Build history of the part. All positions in model axes, mm. Coordinates: 2 decimals unless noted, no trailing zeros. Loops run counter-clockwise (first coordinate to the right, second up) from the corner with the lowest first, then second, coordinate; pieces in that order, holes last.
Item 1: Drill centre lines: line 1 along X through (y, z) = (77, 1.65); line 2 along X through (y, z) = (-5.5, 1); line 3 along X through (y, z) = (26, 1.6). Where is each one in solid material? Low to high.
Item 2: Cut at A-A (z = 1.25). Count the separate pieces of the cut face and the enclosed holes in it, and give its area (3 significant figures).
Item 3: Cut at B-B (x = 2). List the corners of the cut face in (y, z).
Item 4: Flat gauge pins, fed straight in: pin 1 (1 mm diameter, centred on x = 28.5, z = 1.5, fed in from -Y); pin 2 (1 mm diameter, centred on x = -40, z = 0.5, fed in from -Y) (3 decimals); pin 3 (1 mm diameter, centred on x = 48.5, z = 1, fed in from -Y). Where does each tip first touch, or does it go through?
Item 5: Cut at C-C (y = 5). List the corners of the cut face in (x, z).
from build123d import *

# Parameters (mm, degrees)
F0_R     = 1.4
F1_DEPTH = 2
F3_DEPTH = 2.001
F4_R     = 3
F5_R     = 3
F7_DEPTH = 2.001


with BuildPart() as f1:
    # F0 (on Top) → F1 (new body)
    with BuildSketch(Plane.XY):
        Polygon((64.72135955, -47.0228201834), (0, 142.2155100196), (-64.72135955, -47.0228201834), (0, 0), align=None)
        with Locations((-34, 25)):
            Circle(F0_R, mode=Mode.SUBTRACT)
        with Locations((34, 25)):
            Circle(F0_R, mode=Mode.SUBTRACT)
        with Locations((-17, 53.2155100196)):
            Circle(F0_R, mode=Mode.SUBTRACT)
        with Locations((-17, 77.2155100196)):
            Circle(F0_R, mode=Mode.SUBTRACT)
        with Locations((17, 53.2155100196)):
            Circle(F0_R, mode=Mode.SUBTRACT)
        with Locations((17, 77.2155100196)):
            Circle(F0_R, mode=Mode.SUBTRACT)
    extrude(amount=F1_DEPTH)

    # F2 (on face) → F3 (cut, through all)
    with BuildSketch(Plane.XY.offset(2)):
        Polygon((-11.72135955, -5.0228201834), (-46.72135955, -5.0228201834), (-47.4053791086, -7.0228201834), (-14.4741233909, -7.0228201834), align=None)
        Polygon((-12.4188465721, -9.0228201834), (-24.4188465721, -9.0228201834), (-26.4198078873, -10.9094650687), (-15.0155904826, -10.9094650687), align=None)
        Polygon((-23.72135955, -13.0228201834), (-50.72135955, -13.0228201834), (-51.2508899541, -14.5711104259), (-25.8523982474, -14.5711104259), align=None)
        Polygon((-54.6096456252, -17.4572506108), (-55.1764262564, -19.1144565314), (-45.8653729736, -19.1144565314), (-44.7456995673, -17.4572506108), align=None)
        Polygon((-36.183078901, -21.7685099146), (-52.9450522033, -21.7685099146), (-53.5922657988, -23.6608932166), (-38.7877210645, -23.6608932166), align=None)
        Polygon((-57.329058215, -25.4085220489), (-57.8811639638, -27.0228201834), (-51.9252746689, -27.0915274002), (-50.8447687747, -25.4085220489), align=None)
        Polygon((-42.8185183528, -25.398144593), (-49.1967415728, -25.398144593), (-50.3631159663, -27.0228201834), (-44.4640927017, -27.0228201834), align=None)
        Polygon((-34.9575470313, -25.398144593), (-39.6975811287, -25.398144593), (-41.5776334703, -27.0228201834), (-37.1937211406, -27.0228201834), align=None)
        Polygon((-46.72135955, -29.0228201834), (-54.72135955, -29.0228201834), (-55.3310927131, -30.8056147116), (-49.1751657065, -30.8056147116), align=None)
        Polygon((-59.9332226396, -33.0228201834), (-60.6172421983, -35.0228201834), (-58.1569412289, -35.0228201834), (-57.0628715088, -33.0228201834), align=None)
        Polygon((-52.0519517882, -9.9788275021), (-52.6991653837, -11.8712108041), (-38.9741415612, -11.8712108041), (-37.5880427095, -9.9788275021), align=None)
        Polygon((-32.9459308027, -19.1144565314), (-26.3087923894, -19.1144565314), (-24.3671516029, -17.7037719259), (-31.0042900162, -17.7037719259), align=None)
        Polygon((-35.6436006209, -17.440581688), (-43.3317036365, -17.440581688), (-44.5420111982, -19.1144565314), (-37.288930104, -19.1144565314), align=None)
        Polygon((-51.8852360547, -33.0228201834), (-54.9353141808, -33.0228201834), (-56.3333206621, -35.0228201834), (-53.706107908, -35.0228201834), align=None)
        Polygon((-45.4520126634, -33.0228201834), (-50.1858113088, -33.0228201834), (-52.2623182004, -35.0228201834), (-48.2047765043, -35.0228201834), align=None)
        Polygon((-27.9032053004, -9.9788275021), (-35.3451147676, -9.9788275021), (-36.8457930443, -11.8712108041), (-29.7840517014, -11.8712108041), align=None)
        Polygon((24.3671516029, -17.7037719259), (26.3087923894, -19.1144565314), (32.9459308027, -19.1144565314), (31.0042900162, -17.7037719259), align=None)
        Polygon((46.72135955, -29.0228201834), (49.1751657065, -30.8056147116), (55.3310927131, -30.8056147116), (54.72135955, -29.0228201834), align=None)
        Polygon((54.6096456252, -17.4572506108), (44.7456995673, -17.4572506108), (45.8653729736, -19.1144565314), (55.1764262564, -19.1144565314), align=None)
        Polygon((53.5922657988, -23.6608932166), (52.9450522033, -21.7685099146), (36.183078901, -21.7685099146), (38.7877210645, -23.6608932166), align=None)
        Polygon((51.9252746689, -27.0915274002), (57.8811639638, -27.0228201834), (57.329058215, -25.4085220489), (50.8447687747, -25.4085220489), align=None)
        Polygon((51.8852360547, -33.0228201834), (53.706107908, -35.0228201834), (56.3333206621, -35.0228201834), (54.9353141808, -33.0228201834), align=None)
        Polygon((34.9575470313, -25.398144593), (37.1937211406, -27.0228201834), (41.5776334703, -27.0228201834), (39.6975811287, -25.398144593), align=None)
        Polygon((50.1858113088, -33.0228201834), (45.4520126634, -33.0228201834), (48.2047765043, -35.0228201834), (52.2623182004, -35.0228201834), align=None)
        Polygon((26.4198078873, -10.9094650687), (24.4188465721, -9.0228201834), (12.4188465721, -9.0228201834), (15.0155904826, -10.9094650687), align=None)
        Polygon((44.4640927017, -27.0228201834), (50.3631159663, -27.0228201834), (49.1967415728, -25.398144593), (42.8185183528, -25.398144593), align=None)
        Polygon((36.8457930443, -11.8712108041), (35.3451147676, -9.9788275021), (27.9032053004, -9.9788275021), (29.7840517014, -11.8712108041), align=None)
        Polygon((52.0519517882, -9.9788275021), (37.5880427095, -9.9788275021), (38.9741415612, -11.8712108041), (52.6991653837, -11.8712108041), align=None)
        Polygon((43.3317036365, -17.440581688), (35.6436006209, -17.440581688), (37.288930104, -19.1144565314), (44.5420111982, -19.1144565314), align=None)
        Polygon((47.4053791086, -7.0228201834), (46.72135955, -5.0228201834), (11.72135955, -5.0228201834), (14.4741233909, -7.0228201834), align=None)
        Polygon((51.2508899541, -14.5711104259), (50.72135955, -13.0228201834), (23.72135955, -13.0228201834), (25.8523982474, -14.5711104259), align=None)
        Polygon((60.6172421983, -35.0228201834), (59.9332226396, -33.0228201834), (57.0628715088, -33.0228201834), (58.1569412289, -35.0228201834), align=None)
    extrude(amount=-F3_DEPTH, mode=Mode.SUBTRACT)

    # F4
    f4_edges = [f1.edges().sort_by_distance(p)[0] for p in [
        (-64.72136, -47.02282, 1),
    ]]
    fillet(f4_edges, radius=F4_R)

    # F5
    f5_edges = [f1.edges().sort_by_distance(p)[0] for p in [
        (64.72136, -47.02282, 1),
    ]]
    fillet(f5_edges, radius=F5_R)

    # F6 (on face) → F7 (cut, through all)
    with BuildSketch(Plane.XY.offset(2)):
        Polygon((-15.5259804046, 96.8192045811), (0, 81.2669247389), (15.5259804046, 96.8192045811), (0, 142.2155100196), align=None)
    extrude(amount=-F7_DEPTH, mode=Mode.SUBTRACT)


solid = f1.part
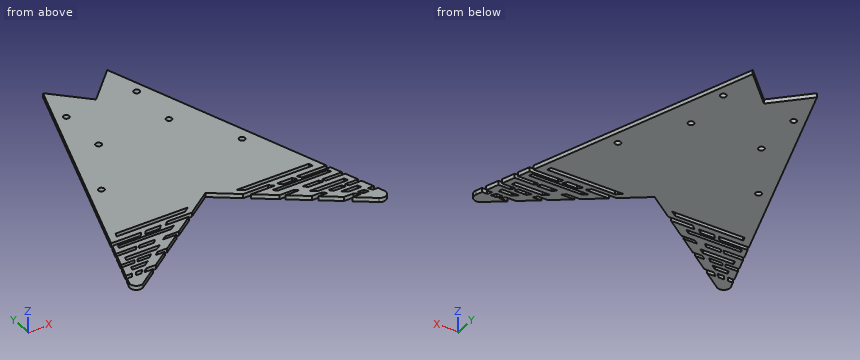
Filled sheet:
1. line 1: x = -22.3 to -18.38, -15.62 to 15.62, 18.38 to 22.3
1. line 2: x = -50.52 to -46.88, -12.38 to -7.57, 7.57 to 12.38, 46.88 to 50.52
1. line 3: x = -39.75 to -34.98, -33.02 to 33.02, 34.98 to 39.75
2. separate pieces: 1
2. enclosed holes: 22
2. area: 7,590 mm2
3. outline: (-1.45, 0) - (83.27, 0) - (83.27, 2) - (-1.45, 2) - close
4. pin 1: stops at y = -21.07
4. pin 2: stops at y = -29.425
4. pin 3: stops at y = -35.6
5. outline: (-46.93, 0) - (46.93, 0) - (46.93, 2) - (-46.93, 2) - close
